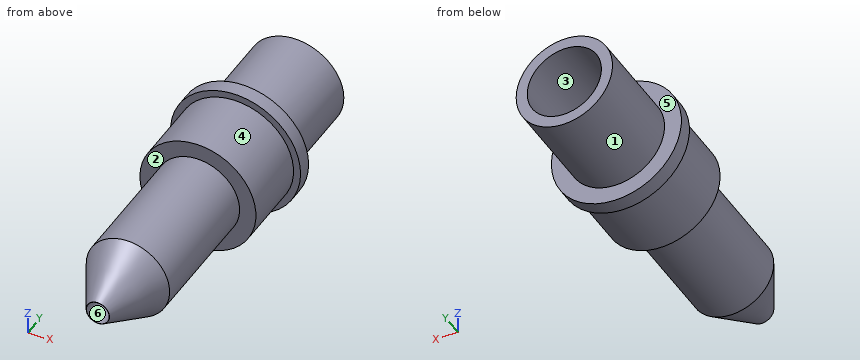
from build123d import *

# Parameters (mm, degrees)
SKETCH1_R           = 10.33
SKETCH1_R_2         = 7.95
BOSS_EXTRUDE1_DEPTH = 20.74
SKETCH2_R           = 13.94
BOSS_EXTRUDE2_DEPTH = 3.2
SKETCH3_R           = 12.44
BOSS_EXTRUDE3_DEPTH = 15
SKETCH4_R           = 8.94
BOSS_EXTRUDE4_DEPTH = 39.88
SKETCH6_R           = 2.45
CUT_EXTRUDE1_DEPTH  = 79.82
SKETCH7_R           = 5.5
CUT_EXTRUDE2_DEPTH  = 46


with BuildPart() as part:
    # Sketch1 → Boss-Extrude1 (new body)
    with BuildSketch(Plane(origin=(0, 0, 0), x_dir=(1, 0, 0), z_dir=(0, 1, 0))):
        Circle(SKETCH1_R)
        Circle(SKETCH1_R_2, mode=Mode.SUBTRACT)
    extrude(amount=BOSS_EXTRUDE1_DEPTH)

    # Sketch2 → Boss-Extrude2 (add)
    with BuildSketch(Plane.XZ):
        Circle(SKETCH2_R)
    extrude(amount=BOSS_EXTRUDE2_DEPTH)

    # Sketch3 → Boss-Extrude3 (add)
    with BuildSketch(Plane(origin=(0, -3.2, 0), x_dir=(-1, 0, 0), z_dir=(0, -1, 0))):
        Circle(SKETCH3_R)
    extrude(amount=BOSS_EXTRUDE3_DEPTH)

    # Sketch4 → Boss-Extrude4 (add)
    with BuildSketch(Plane(origin=(0, -18.2, 0), x_dir=(-1, 0, 0), z_dir=(0, -1, 0))):
        Circle(SKETCH4_R)
    extrude(amount=BOSS_EXTRUDE4_DEPTH)

    # Sketch5 → Cut-Revolve1 (revolve, cut)
    with BuildSketch(Plane(origin=(0, 0, 0), x_dir=(0, 0, -1), z_dir=(1, 0, 0))):
        Polygon((8.94, -46.08), (2.5, -58.08), (8.94, -58.08), align=None)
    revolve(axis=Axis((0, -58.08, 0), (0, 1, 0)), mode=Mode.SUBTRACT)

    # Sketch6 → Cut-Extrude1 (cut, through all)
    with BuildSketch(Plane.XZ.offset(58.08)):
        Circle(SKETCH6_R)
    extrude(amount=-CUT_EXTRUDE1_DEPTH, mode=Mode.SUBTRACT)

    # Sketch7 → Cut-Extrude2 (cut)
    with BuildSketch(Plane(origin=(0, 0, 0), x_dir=(1, 0, 0), z_dir=(0, 1, 0))):
        Circle(SKETCH7_R)
    extrude(amount=-CUT_EXTRUDE2_DEPTH, mode=Mode.SUBTRACT)


solid = part.part
The model under review builds one solid part; all positions refer to its coordinate system, in mm. Face numbers are marked on the shaded views. A direction names the side the tool comes from. Give positions to 0.01 mm unless a question says otherwise; leave off trailing zeros. Write each loop counter-clockwise with the first axis right and the second up, starting at its lowest first coordinate (ties: lowest second). Pieces come first, ordered by that corner, then holes. Notation, with made-up numbers: M 50,17.25 L 96,17.25 A8 ccw 96,24.25 Z; hole C 7.5,49 d6. An arc over 180 degrees is marked long. One line per question, with ' | ' between items. Start each with the question number.
Item 1: We need section D-D on y = -48. Write out the cut boundary in (x, z), plus the area to 3 significant figures.
Item 2: For pin 1 (4 mm diameter, centred on x = 7, y = -17, fed in from -Z); pin 2 (8 mm diameter, centred on y = -19, z = -6, fed in from -X); pin 3 (1.5 mm diameter, centred on x = -11, z = 2.5, fed in from +Y), all flat-tipped, find the tip position at first contact; note any pin that passes through.
Item 3: Wall thickness on line 1 (X direction, y = -17.5, z = 0); line 2 (X direction, y = 8.5, z = 0.25): over which ranges is each line inside the solid? List them lowest first. Write a range as from..to.
Item 4: Draft analysis for pull direction Z (two halves, no side actions). For the marked faces 1, 2 and 3, state which applies: released by +Z, released by -Z, zero draft, split by the parting line, or undercut.
Item 5: We need section C-C on y = -15.5. Write out the cut boundary in (x, z).
Item 6: For the marked faces 4, 5 and 6, list the 3-axis set-ups (+Z, -Z, +X, -X, +Y, -Y) from which the entire face can be reached by the end or side of a thin tool; tool diameter is ignored.
Results found:
1) outline: C 0,0 d15.82; hole C 0,0 d4.9 | area: 178 mm2
2) pin 1: stops at z = -11.39 | pin 2: stops at x = -12.26 | pin 3: stops at y = 0
3) line 1: x = -12.44..-5.5, 5.5..12.44 | line 2: x = -10.33..-7.95, 7.95..10.33
4) face 1: split by the parting line | face 2: zero draft | face 3: undercut
5) outline: C 0,0 d24.88; hole C 0,0 d11
6) face 4: -Y | face 5: +Y | face 6: +Y, -Y
